Geometry check sheet. Reference: the model listing, model coordinates, mm. A direction names the side the tool comes from. Round coordinates to 2 decimals unless told otherwise and drop trailing zeros. Write each loop counter-clockwise with the first axis right and the second up, starting at its lowest first coordinate (ties: lowest second). Pieces come first, ordered by that corner, then holes.
Item 1: Access from +Z, -Z, +X, -X, +Y, -Y to the whole of each face (thin tool, end or side, straight path). Record for faces 5 (the face through (1.62, -0.67, 33.37)), 6 (the face through (-1.67, 0.53, -33.37)), 7 (the face through (-1.4, 1.4, -38.1)).
Item 2: Draft check along X on faces 1 (the face through (0, 0, 28.575)), 2 (the face through (-1.4, 1.4, 38.1)), 3 (the face through (-1.5, 2.8, -0.5)), 4 (the face through (0, 0, -28.575)). Enter one of: pulls with the +X half, pulls with the -X half, needs draft (parallel to the pull), parting line crosses it, or undercut.
Item 3: Depth check by flat-ended pin: P1, Ø3, axis at x = 1, y = 1, coming from the +Z side; P2, Ø3, axis at x = 0, y = 0, coming from the -Z side (3 decimals); P3, Ø1, axis at x = -1, z = 18.5, coming from the +Y side; P4, Ø3, axis at x = 0, y = 0, coming from the +Z side (3 decimals). Enter the tip coordinate at first touch or a pass-through.
Item 4: Scan lines: probe 1 along Y at (x, z) = (0, -31.5) (3 decimals); probe 2 along Z at (x, y) = (-0.5, 1.25) (3 decimals); probe 3 along Y at (x, z) = (-0.5, -30). Record each from-to range of solid material in increasing order.
Item 5: Cross-section at A-A (x = 0). Enter the section's corners in (y, z) (3 decimals).
Item 6: Cross-section at B-B (z = 6.5). Enter the section's corners in (x, y) (3 decimals), then the cut area to 3 significant figures.
from build123d import *

# Parameters (mm, degrees)
BOSS_EXTRUDE1_START = 38.1
SKETCH13_R          = 1.7526
BOSS_EXTRUDE1_DEPTH = 9.525
CIRPATTERN1_COUNT   = 2
CIRPATTERN1_ANGLE   = 180
EXTRUDE1_DEPTH      = 38.1
EXTRUDE1_DEPTH_BACK = 38.1
SKETCH1_R           = 3.175


with BuildPart() as part:
    # Sketch13 → Boss-Extrude1 (new body)
    with BuildSketch(Plane.XY.offset(BOSS_EXTRUDE1_START)):
        Circle(SKETCH13_R)
    extrude(amount=-BOSS_EXTRUDE1_DEPTH)

    # Boss-Extrude2 cone 1 section (through the dimple's axis) → Boss-Extrude2 (revolve)
    with BuildSketch(Plane(origin=(0, 0, 38.1), x_dir=(0, -1, 0), z_dir=(1, 0, 0))):
        Polygon((0, 0), (1.8288, 0), (0, 1.8288), align=None)
    revolve(axis=Axis((0, 0, 38.1), (0, 0, -1)))


with BuildPart() as cirpattern1_1:
    # CirPattern1: pattern copy
    add(part.part.rotate(Axis((0, 3.175, 0), (0, -1, 0)), 1 * CIRPATTERN1_ANGLE / (CIRPATTERN1_COUNT - 1)))


with BuildPart() as body_3:
    # Sketch1 → Extrude1 (new, two sides: drawn at the far end of the back side and taken through both)
    with BuildSketch(Plane.XY.offset(-EXTRUDE1_DEPTH_BACK)):
        with Locations(Location((0, 0, 0), (0, 0, 180))):
            Circle(SKETCH1_R)
    extrude(amount=EXTRUDE1_DEPTH + EXTRUDE1_DEPTH_BACK)

    # Combine1: cut CirPattern1_1, part
    add(cirpattern1_1.part, mode=Mode.SUBTRACT)
    add(part.part, mode=Mode.SUBTRACT)


solid = body_3.part
Resolved:
1. face 5: +Z
1. face 6: -Z
1. face 7: -Z, +X, -X, +Y, -Y
2. face 1: undercut
2. face 2: needs draft
2. face 3: parting line crosses it
2. face 4: undercut
3. P1: stops at z = 38.1
3. P2: stops at z = -28.575
3. P3: stops at y = 3.14
3. P4: stops at z = 28.575
4. probe 1: y = -3.175 to -1.753, 1.753 to 3.175
4. probe 2: z = -28.575 to 28.575
4. probe 3: y = -3.14 to -1.68, 1.68 to 3.14
5. outline: (-3.175, -38.1) - (-1.829, -38.1) - (-1.753, -38.024) - (-1.753, -28.575) - (1.753, -28.575) - (1.753, -38.024) - (1.829, -38.1) - (3.175, -38.1) - (3.175, 38.1) - (1.829, 38.1) - (1.753, 38.024) - (1.753, 28.575) - (-1.753, 28.575) - (-1.753, 38.024) - (-1.829, 38.1) - (-3.175, 38.1) - close
6. outline: circle Ø6.35 at (0, 0)
6. area: 31.7 mm2
